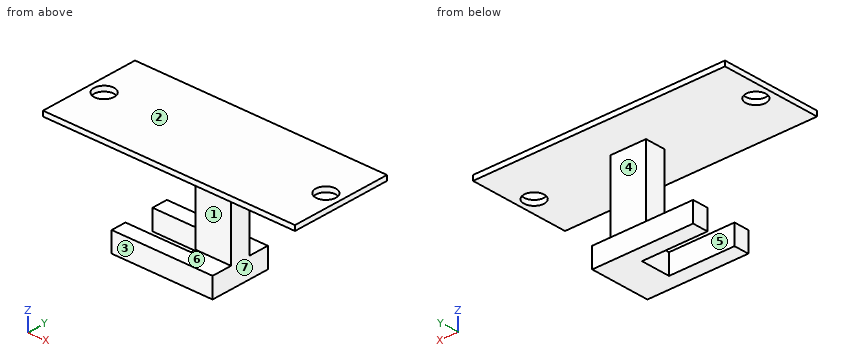
Autodesk Fusion 360 part; units mm, degrees
sketch "Sketch1" plane through (0, 0, 0) normal (0, 0, 1) x (1, 0, 0)
  line L0 (0, 0) -> (50, 0)
  line L1 (50, 0) -> (50, 20)
  line L2 (50, 20) -> (0, 20)
  line L3 (0, 20) -> (0, 0)
  dimension "d1" = 50
  dimension "d2" = 20
extrude "Extrude1" add sketch "Sketch1" along normal blind 1
sketch "Sketch2" plane through (0, 0, 1) normal (0, 0, 1) x (-1, 0, 0)
  line L0 (0, -20) -> (0, 0)
  line L1 (0, 0) -> (-50, 0)
  line L2 (-50, 0) -> (-50, -20)
  line L3 (-50, -20) -> (0, -20)
  circle A0 centre (-3, -10) radius 2
  circle A1 centre (-47, -10) radius 2
  dimension "d8" = 4
  dimension "d19" = 4
extrude "Extrude2" cut sketch "Sketch2" against normal blind 7 contours A0 | A1
sketch "Sketch3" plane through (0, 0, 0) normal (0, 0, -1) x (1, 0, 0)
  circle A0 centre (3, -10) radius 2
  line L0 (0, 0) -> (0, -20)
  line L1 (0, -20) -> (50, -20)
  line L2 (50, -20) -> (50, 0)
  line L3 (50, 0) -> (0, 0)
  line L4 (22.9728, -8) -> (30, -8)
  line L5 (30, -8) -> (30, -12)
  line L6 (30, -12) -> (22.9728, -12)
  line L7 (22.9728, -12) -> (22.9728, -8)
  circle A1 centre (46, -10) radius 2
  circle A2 centre (47, -10) radius 2
extrude "Extrude3" add sketch "Sketch3" along normal blind 21 contours L4 L5 L6 L7
sketch "Sketch6" plane through (0, 8, 0) normal (0, -1, 0) x (1, 0, 0)
  line L0 (30, 0) -> (22.9728, 0)
  line L1 (22.9728, 0) -> (22.9728, -21)
  line L2 (22.9728, -21) -> (30, -21)
  line L3 (30, -21) -> (30, 0)
  line L4 (22.9728, -21) -> (30, -21)
  line L5 (30, -21) -> (30, -17)
  line L6 (30, -17) -> (22.9728, -17)
  line L7 (22.9728, -17) -> (22.9728, -21)
extrude "Extrude4" add sketch "Sketch6" along normal blind 4 contours L1 L2 L3 L4 L5 L6 L7
extrude "Extrude5" add sketch "Sketch6" against normal blind 8 contours L1 L2 L3 L4 L5 L6 L7
sketch "Sketch7" plane through (22.9728, 0, 0) normal (-1, 0, 0) x (0, -1, 0)
  line L0 (-16, -21) -> (-4, -21)
  line L1 (-4, -21) -> (-4, -17)
  line L2 (-4, -17) -> (-8, -17)
  line L3 (-8, -17) -> (-8, 0)
  line L4 (-8, 0) -> (-12, 0)
  line L5 (-12, 0) -> (-12, -17)
  line L6 (-12, -17) -> (-16, -17)
  line L7 (-16, -17) -> (-16, -21)
  line L8 (-16, -17) -> (-12.8799, -17)
  line L9 (-12.8799, -17) -> (-12.8799, -21)
  line L10 (-12.8799, -21) -> (-16, -21)
  line L11 (-16, -21) -> (-16, -17)
  line L12 (-4, -21) -> (-7, -21)
  line L13 (-7, -21) -> (-7, -17)
  line L14 (-7, -17) -> (-4, -17)
  line L15 (-4, -17) -> (-4, -21)
extrude "Extrude6" add sketch "Sketch7" along normal blind 13 contours L0 L6 L7 L8 L9 L10 L11 | L0 L1 L2 L12 L13 L14 L15
Here's how the part is built. I have some questions about the finished solid (model axes, mm). Face numbers are marked on the shaded views. A direction names the side the tool comes from. Give positions to 0.01 mm unless a question says otherwise; leave off trailing zeros. Write each loop counter-clockwise with the first axis right and the second up, starting at its lowest first coordinate (ties: lowest second). Pieces come first, ordered by that corner, then holes.
(1) Imagine slicing it at D-D, the plane y = 18. Write out the boundary of the cut face in (x, z), and give its area (3 significant figures).
Output values:
outline: (0, 0) - (50, 0) - (50, 1) - (0, 1) - close
area: 50.0 mm2
(2) Will these pins go through, and if not, where does the flat tip stop? pin 1 (3.5 mm diameter, centred on y = 7.5, z = -6, fed in from +X); pin 2 (2 mm diameter, centred on x = 10, z = -2.5, fed in from +Y); pin 3 (7.5 mm diameter, centred on x = 26.5, z = -8.5, fed in from +Y); pin 4 (6.5 mm diameter, centred on y = 11, z = -11.5, fed in from -X).
Output values:
pin 1: stops at x = 30
pin 2: passes through
pin 3: stops at y = 12
pin 4: stops at x = 22.97
(3) Thinking about a two-plate mould opening in Z: for the marked faces 1, 2 and 3, which applies, pulls with the +Z half, pulls with the -Z half, needs draft (parallel to the pull), parting line crosses it, or undercut?
Output values:
face 1: undercut
face 2: pulls with the +Z half
face 3: needs draft
(4) Imagine slicing it at C-C, the plane x = 4. Write out the boundary of the cut face in (y, z), and give its area (3 significant figures).
Output values:
outline: (0, 0) - (8.27, 0) - (8.27, 1) - (0, 1) - close; (11.73, 0) - (20, 0) - (20, 1) - (11.73, 1) - close
area: 16.5 mm2
(5) If I drill on L1, parallel to X at y = 10, z = 0.7; L2, parallel to Z at x = 22.5, y = 5.5; L3, parallel to Y at x = 18, z = -18.75, over which ranges is the centre line in solid material (lowest first)?
Output values:
L1: x = 0 to 1, 5 to 45, 49 to 50
L2: z = -21 to -17, 0 to 1
L3: y = 4 to 7, 12.88 to 16
(6) Imagine slicing it at B-B, the plane x = 47. Write out the boundary of the cut face in (y, z).
Output values:
outline: (0, 0) - (8, 0) - (8, 1) - (0, 1) - close; (12, 0) - (20, 0) - (20, 1) - (12, 1) - close
(7) Imagine slicing it at A-A, the plane y = 10. Write out the boundary of the cut face in (x, z).
Output values:
outline: (0, 0) - (1, 0) - (1, 1) - (0, 1) - close; (5, 0) - (22.97, 0) - (22.97, -21) - (30, -21) - (30, 0) - (45, 0) - (45, 1) - (5, 1) - close; (49, 0) - (50, 0) - (50, 1) - (49, 1) - close
(8) On a 3-axis mill with a long thin cutter (end or side, diameter ignored), from which of +Z, -Z, +X, -X, +Y, -Y can I reach the whole of each face in a straight line? I mean the marked faces 4, 5, 6 and 7. Say none if no direction works.
Output values:
face 4: +X, -X, +Y
face 5: -Z, -X
face 6: +X, -X, -Y
face 7: -Z, +X, +Y, -Y
